```python
from build123d import *

# Parameters (mm, degrees)
PAD_DEPTH       = 15
SKETCH001_W     = 15
SKETCH001_H     = 15
POCKET_DEPTH    = 12
SKETCH002_R     = 2.5
POCKET001_DEPTH = 5
SKETCH003_R     = 2.5
POCKET002_DEPTH = 19
CHAMFER_SIZE    = 2


with BuildPart() as part:
    # Sketch → Pad (new body)
    with BuildSketch(Plane.XY):
        Polygon((-15, 15), (-12, 15), (0, 3), (0, 0), (-15, 0), align=None)
    extrude(amount=PAD_DEPTH)

    # Sketch001 → Pocket (cut)
    with BuildSketch(Plane.XY.offset(1.5)):
        with Locations((-4.5, 10.5)):
            Rectangle(SKETCH001_W, SKETCH001_H)
    extrude(amount=POCKET_DEPTH, mode=Mode.SUBTRACT)

    # Sketch002 → Pocket001 (cut)
    with BuildSketch(Plane.XZ):
        with Locations((-4.9995, 7.5)):
            Circle(SKETCH002_R)
    extrude(amount=-POCKET001_DEPTH, mode=Mode.SUBTRACT)

    # Sketch003 → Pocket002 (cut)
    with BuildSketch(Plane.YZ):
        with Locations((9.999, 7.5)):
            Circle(SKETCH003_R)
    extrude(amount=-POCKET002_DEPTH, mode=Mode.SUBTRACT)

    # Chamfer
    chamfer_edges = [part.edges().sort_by_distance(p)[0] for p in [
        (-15, 0, 7.5),
    ]]
    chamfer(chamfer_edges, length=CHAMFER_SIZE)


solid = part.part
```
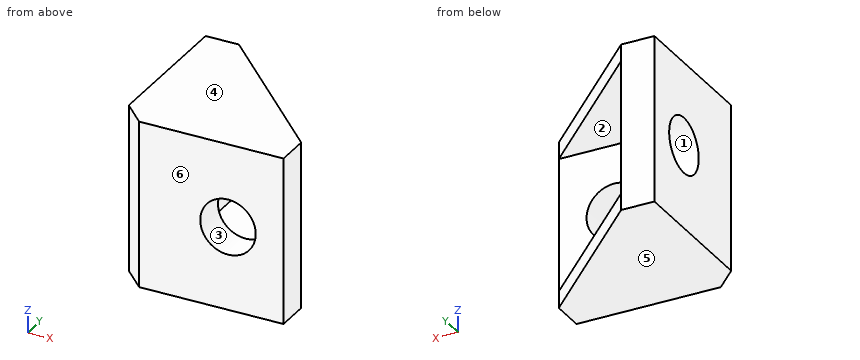
For this review, take the finished solid that the model builds, in its own axes (mm). Face numbers are marked on the shaded views. A direction names the side the tool comes from. Give positions to 0.01 mm unless a question says otherwise; leave off trailing zeros. Write each loop counter-clockwise with the first axis right and the second up, starting at its lowest first coordinate (ties: lowest second). Pieces come first, ordered by that corner, then holes. Notation, with made-up numbers: M -9.5,58 L 13.5,58 A19 ccw 13.5,67 Z; hole C 40,19.25 d4. An arc over 180 degrees is marked long. Answer as a JSON object with one key per item and string values. Group by question number.
Item 1: For probe 1 along Z at (x, y) = (-10, 11.5); probe 2 along X at (y, z) = (7, 7.25); probe 3 along Y at (x, z) = (-11.5, 9), list the stretches that pass through material, from the lowest coordinate up. Write a range as [from, to].
Item 2: Consider section C-C on y = 6.5. Write out the cut boundary in (x, z), plus the area to 3 significant figures.
Item 3: Tool access review of the marked faces 1 and 2: name each direction out of +Z, -Z, +X, -X, +Y, -Y from which nothing blocks a thin tool from reaching the whole face with its end or side.
Item 4: Consider section B-B on x = -5. Write out the cut boundary in (y, z), plus the area to 3 significant figures.
Item 5: Consider section A-A on z = 7.5. Write out the cut boundary in (x, y).
Item 6: For pin 1 Ø3 at (x, z) = (-3, 11.5) entering from +Y; pin 2 Ø4 at (x, z) = (-5, 7.5) entering from +Y; pin 3 Ø6 at (y, z) = (9.999, 7.5) entering from -X, all flat-tipped, find the tip position at first contact; note any pin that passes through.
Item 7: Draft analysis for pull direction Z (two halves, no side actions). For the marked faces 3, 4, 5 and 6, state which applies: +Z half, -Z half, draft (parallel to the pull), parting line (faces both ways), or undercut.
Item 8: Consider section D-D on x = -12.75. Write out the cut boundary in (y, z).
Check result:
{
 "1": {"probe 1": "z = [0, 1.5], [13.5, 15]", "probe 2": "x = [-15, -12]", "probe 3": "y = [0, 3]"},
 "2": {"outline": "M -15,0 L -3.5,0 L -3.5,1.5 L -12,1.5 L -12,13.5 L -3.5,13.5 L -3.5,15 L -15,15 Z", "area": "70.5 mm^2"},
 "3": {"face 1": "+X, -X", "face 2": "+X, +Y"},
 "4": {"outline": "M 0,0 L 8,0 L 8,1.5 L 3,1.5 L 3,5 L 0,5 Z; M 0,10 L 3,10 L 3,13.5 L 8,13.5 L 8,15 L 0,15 Z", "area": "45.0 mm^2"},
 "5": {"outline": "M -15,2 L -13,0 L -7.5,0 L -7.5,3 L -12,3 L -12,7.5 L -15,7.5 Z; M -15,12.5 L -12,12.5 L -12,15 L -15,15 Z; M -2.5,0 L 0,0 L 0,3 L -2.5,3 Z"},
 "6": {"pin 1": "stops at y = 3", "pin 2": "passes through", "pin 3": "stops at x = -15"},
 "7": {"face 3": "undercut", "face 4": "+Z half", "face 5": "-Z half", "face 6": "draft"},
 "8": {"outline": "M 0,0 L 15,0 L 15,15 L 0,15 Z; hole C 10,7.5 d5"}
}
